```python
from build123d import *

# Parameters (mm, degrees)
SKETCH1_W            = 129.0828
SKETCH1_H            = 88.5698
BOSS_EXTRUDE1_DEPTH  = 3.175
SKETCH3_W            = 47.9044
SKETCH3_H            = 79.0448
CUT_EXTRUDE1_DEPTH   = 4.175
FILLET1_R            = 3.175
SKETCH5_W            = 38.1
SKETCH5_H            = 2.794
SKETCH5_W_2          = 2.794
SKETCH5_H_2          = 50.8
BOSS_EXTRUDE2_DEPTH  = 3.175
FILLET2_R            = 1.5875
FILLET2_OF_MIRROR1_R = 1.5875
M3_CLEARANCE_HOLE1_D = 3.4


with BuildPart() as part:
    # Sketch1 → Boss-Extrude1 (new body)
    with BuildSketch(Plane(origin=(0, 0, 0), x_dir=(1, 0, 0), z_dir=(0, 1, 0))):
        Rectangle(SKETCH1_W, SKETCH1_H)
    extrude(amount=BOSS_EXTRUDE1_DEPTH)

    # Sketch3 → Cut-Extrude1 (cut, through all)
    with BuildSketch(Plane.XZ):
        with Locations((-31.2547, 0)):
            Rectangle(SKETCH3_W, SKETCH3_H)
        with Locations((31.2547, 0)):
            Rectangle(SKETCH3_W, SKETCH3_H)
    extrude(amount=-CUT_EXTRUDE1_DEPTH, mode=Mode.SUBTRACT)

    # Fillet1
    fillet1_edges = [part.edges().sort_by_distance(p)[0] for p in [
        (-7.3025, 1.5875, -39.5224),
        (-55.2069, 1.5875, -39.5224),
        (-55.2069, 1.5875, 39.5224),
        (-7.3025, 1.5875, 39.5224),
        (55.2069, 1.5875, -39.5224),
        (7.3025, 1.5875, -39.5224),
        (7.3025, 1.5875, 39.5224),
        (55.2069, 1.5875, 39.5224),
        (-64.5414, 1.5875, -44.2849),
        (64.5414, 1.5875, -44.2849),
        (64.5414, 1.5875, 44.2849),
        (-64.5414, 1.5875, 44.2849),
    ]]
    fillet(fillet1_edges, radius=FILLET1_R)

    # Sketch5 → Boss-Extrude2 (add)
    with BuildSketch(Plane.XZ):
        with Locations((-31.2547, 42.8879)):
            Rectangle(SKETCH5_W, SKETCH5_H)
        with Locations((-60.1599, 0)):
            Rectangle(SKETCH5_W_2, SKETCH5_H_2)
        with Locations((-31.2547, -42.8879)):
            Rectangle(SKETCH5_W, SKETCH5_H)
    boss_extrude2 = extrude(amount=BOSS_EXTRUDE2_DEPTH)

    # Fillet2
    fillet2_edges = [part.edges().sort_by_distance(p)[0] for p in [
        (-50.3047, 0, 42.8879),
        (-12.2047, 0, 42.8879),
        (-61.5569, 0, 0),
        (-60.1599, 0, -25.4),
        (-60.1599, 0, 25.4),
        (-50.3047, 0, -42.8879),
        (-12.2047, 0, -42.8879),
    ]]
    fillet(fillet2_edges, radius=FILLET2_R)

    # Mirror1: Boss-Extrude2 across plane
    add(boss_extrude2.mirror(Plane(origin=(0, 0, 0), x_dir=(0, 0, 1), z_dir=(1, 0, 0))))

    # Fillet2 of Mirror1
    fillet2_of_mirror1_edges = [part.edges().sort_by_distance(p)[0] for p in [
        (50.3047, 0, 42.8879),
        (12.2047, 0, 42.8879),
        (61.5569, 0, 0),
        (60.1599, 0, -25.4),
        (60.1599, 0, 25.4),
        (50.3047, 0, -42.8879),
        (12.2047, 0, -42.8879),
    ]]
    fillet(fillet2_of_mirror1_edges, radius=FILLET2_OF_MIRROR1_R)

    # M3 Clearance Hole1 (through all)
    with Locations(Plane(origin=(0, 3.175, 0), x_dir=(1, 0, 0), z_dir=(0, 1, 0))):
        with Locations((0, 31.75), (0, -31.75)):
            Hole(M3_CLEARANCE_HOLE1_D / 2)


solid = part.part
```
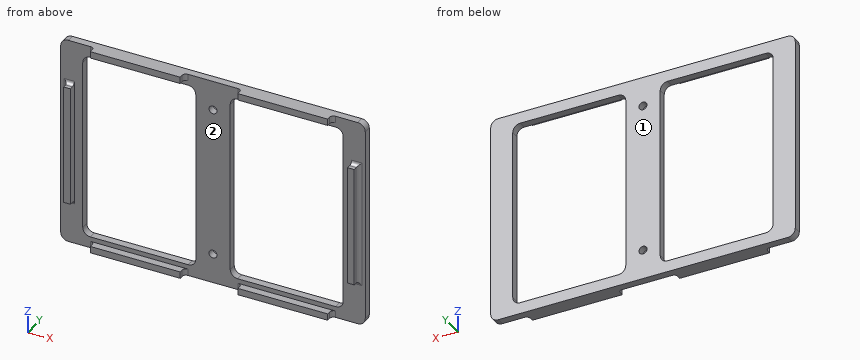
Verification items for the finished model (mm, model axes). Face numbers are marked on the shaded views. Round coordinates to 2 decimals unless told otherwise and drop trailing zeros. Write each loop counter-clockwise with the first axis right and the second up, starting at its lowest first coordinate (ties: lowest second). Pieces come first, ordered by that corner, then holes.
1. Section check C-C on z = 18.5. Enter the section's corners in (x, y) (1 decimal), plus the area to 3 significant figures.
2. Section check A-A on x = 0. Enter the section's corners in (y, z) (3 decimals).
3. Draft check along Z on the marked faces 1 and 2. Enter one of: +Z half, -Z half, draft (parallel to the pull), parting line (faces both ways), or undercut.
4. Scan lines: L1, parallel to X at y = 1.5, z = 31.75; L2, parallel to Z at x = 0, y = 1.05; L3, parallel to X at y = 2.25, z = 17.5. Record each from-to range of solid material in increasing order.
5. Gauge pin test, flat ends, axial feed: P1, Ø0.8, axis at y = -2, z = -43, coming from the -X side; P2, Ø1.7, axis at y = -2, z = 5, coming from the -X side; P3, Ø1.3, axis at y = -2, z = 8.5, coming from the +X side; P4, Ø3.5, axis at y = -1.5, z = -9, coming from the -X side. Record the tip position at first contact, or that the pin passes through.
6. Section check B-B on z = 31.75. Enter the section's corners in (x, y) (1 decimal).
Answer:
1. outline: (-64.5, 0) - (-63.1, 0) arc R1.6 cw to (-61.6, -1.6) - (-61.6, -3.2) - (-58.8, -3.2) - (-58.8, 0) - (-55.2, 0) - (-55.2, 3.2) - (-64.5, 3.2) - close; (-7.3, 0) - (7.3, 0) - (7.3, 3.2) - (-7.3, 3.2) - close; (55.2, 0) - (58.8, 0) - (58.8, -3.2) - (61.6, -3.2) - (61.6, -1.6) arc R1.6 cw to (63.1, 0) - (64.5, 0) - (64.5, 3.2) - (55.2, 3.2) - close
1. area: 124 mm2
2. outline: (0, -44.285) - (3.175, -44.285) - (3.175, -33.45) - (0, -33.45) - close; (0, -30.05) - (3.175, -30.05) - (3.175, 30.05) - (0, 30.05) - close; (0, 33.45) - (3.175, 33.45) - (3.175, 44.285) - (0, 44.285) - close
3. face 1: draft
3. face 2: undercut
4. L1: x = -64.54 to -55.21, -7.3 to -1.7, 1.7 to 7.3, 55.21 to 64.54
4. L2: z = -44.28 to -33.45, -30.05 to 30.05, 33.45 to 44.28
4. L3: x = -64.54 to -55.21, -7.3 to 7.3, 55.21 to 64.54
5. P1: stops at x = -50.3
5. P2: stops at x = -61.62
5. P3: stops at x = 61.57
5. P4: stops at x = -64.54
6. outline: (-64.5, 0) - (-55.2, 0) - (-55.2, 3.2) - (-64.5, 3.2) - close; (-7.3, 0) - (-1.7, 0) - (-1.7, 3.2) - (-7.3, 3.2) - close; (1.7, 0) - (7.3, 0) - (7.3, 3.2) - (1.7, 3.2) - close; (55.2, 0) - (64.5, 0) - (64.5, 3.2) - (55.2, 3.2) - close
